Autodesk Inventor part; units mm, degrees
ref_plane "YZ Plane" through (0, 0, 0) normal (1, 0, 0) x (0, 1, 0)
ref_plane "XZ Plane" through (0, 0, 0) normal (0, 1, 0) x (-1, 0, 0)
ref_plane "XY Plane" through (0, 0, 0) normal (0, 0, 1) x (1, 0, 0)
ref_plane "작업 평면1" through (0, 0, 0) normal (0, 0, 1) x (1, 0, 0)
sketch "스케치1" plane through (0, 0, 0) normal (0, 0, 1) x (1, 0, 0)
  line L0 (-85.3, -15) -> (-85.3, -11.5)
  line L1 (-85.3, -15) -> (-79.3, -20.1)
  line L2 (-79.3, -20.1) -> (-26.2, -20.1)
  line L3 (-26.2, -20.1) -> (-20.2, -15)
  line L4 (-20.2, -15) -> (-20.2, 15)
  line L5 (-20.2, 15) -> (-26.2, 20.1)
  line L6 (-26.2, 20.1) -> (-79.3, 20.1)
  line L7 (-79.3, 20.1) -> (-85.3, 15)
  line L8 (-85.3, 11.5) -> (-85.3, 15)
  arc A0 (-82.3, 14.5) -> (-85.3, 11.5) centre (-82.3, 11.5) ccw
  line L9 (-28.8, 14.5) -> (-82.3, 14.5)
  arc A1 (-25.8, 11.5) -> (-28.8, 14.5) centre (-28.8, 11.5) ccw
  line L10 (-25.8, -11.5) -> (-25.8, 11.5)
  arc A2 (-28.8, -14.5) -> (-25.8, -11.5) centre (-28.8, -11.5) ccw
  line L11 (-82.3, -14.5) -> (-28.8, -14.5)
  arc A3 (-85.3, -11.5) -> (-82.3, -14.5) centre (-82.3, -11.5) ccw
  circle A4 centre (-74.8, 17.3) radius 1.35
  circle A5 centre (-52.8, 17.3) radius 1.35
  circle A6 centre (-30.8, 17.3) radius 1.35
  circle A7 centre (-23, 11) radius 1.35
  circle A8 centre (-74.8, -17.3) radius 1.35
  circle A9 centre (-52.8, -17.3) radius 1.35
  circle A10 centre (-30.8, -17.3) radius 1.35
  circle A11 centre (-23, -11) radius 1.35
  line L12 (-15, 14.5) -> (-11.5, 14.5)
  line L13 (-15, 14.5) -> (-20.1, 8.5)
  line L14 (-20.1, 8.5) -> (-20.1, -44.6)
  line L15 (-20.1, -44.6) -> (-15, -50.6)
  line L16 (-15, -50.6) -> (15, -50.6)
  line L17 (15, -50.6) -> (20.1, -44.6)
  line L18 (20.1, -44.6) -> (20.1, 8.5)
  line L19 (20.1, 8.5) -> (15, 14.5)
  line L20 (11.5, 14.5) -> (15, 14.5)
  arc A12 (14.5, 11.5) -> (11.5, 14.5) centre (11.5, 11.5) ccw
  line L21 (14.5, -42) -> (14.5, 11.5)
  arc A13 (11.5, -45) -> (14.5, -42) centre (11.5, -42) ccw
  line L22 (-11.5, -45) -> (11.5, -45)
  arc A14 (-14.5, -42) -> (-11.5, -45) centre (-11.5, -42) ccw
  line L23 (-14.5, 11.5) -> (-14.5, -42)
  arc A15 (-11.5, 14.5) -> (-14.5, 11.5) centre (-11.5, 11.5) ccw
  circle A16 centre (17.3, 4) radius 1.35
  circle A17 centre (17.3, -18) radius 1.35
  circle A18 centre (17.3, -40) radius 1.35
  circle A19 centre (11, -47.8) radius 1.35
  circle A20 centre (-17.3, 4) radius 1.35
  circle A21 centre (-17.3, -18) radius 1.35
  circle A22 centre (-17.3, -40) radius 1.35
  circle A23 centre (-11, -47.8) radius 1.35
  arc A24 (-14.6, -42) -> (-11.5, -45.1) centre (-11.5, -42) ccw
  line L24 (-11.5, -45.1) -> (11.5, -45.1)
  arc A25 (11.5, -45.1) -> (14.6, -42) centre (11.5, -42) ccw
  line L25 (14.6, -42) -> (14.6, 11.5)
  arc A26 (14.6, 11.5) -> (12.5954, 14.4) centre (11.5, 11.5) ccw
  line L26 (12.5954, 14.4) -> (14.9538, 14.4)
  line L27 (14.9538, 14.4) -> (20, 8.4632)
  line L28 (20, 8.4632) -> (20, -44.5632)
  line L29 (14.9538, -50.5) -> (-14.9538, -50.5)
  line L30 (-14.6, 11.5) -> (-14.6, -42)
  arc A27 (-25.7, 11.5) -> (-28.8, 14.6) centre (-28.8, 11.5) ccw
  line L31 (-28.8, 14.6) -> (-82.3, 14.6)
  arc A28 (-82.3, 14.6) -> (-85.2, 12.5954) centre (-82.3, 11.5) ccw
  line L32 (-85.2, 12.5954) -> (-85.2, 14.9538)
  line L33 (-85.2, 14.9538) -> (-79.2632, 20)
  line L34 (-79.2632, 20) -> (-26.2368, 20)
  line L35 (-20.3, -14.9538) -> (-26.2368, -20)
  line L36 (-26.2368, -20) -> (-79.2632, -20)
  line L37 (-79.2632, -20) -> (-85.2, -14.9538)
  line L38 (-85.2, -14.9538) -> (-85.2, -12.5954)
  arc A29 (-85.2, -12.5954) -> (-82.3, -14.6) centre (-82.3, -11.5) ccw
  line L39 (-82.3, -14.6) -> (-28.8, -14.6)
  arc A30 (-28.8, -14.6) -> (-25.7, -11.5) centre (-28.8, -11.5) ccw
  line L40 (-25.7, -11.5) -> (-25.7, 11.5)
  line L41 (-14.6, 15.6629) -> (-14.6, -30)
  circle A31 centre (-23, -11) radius 1.35
  circle A32 centre (-23, 11) radius 1.35
  circle A33 centre (-17.3, -18) radius 1.35
  circle A34 centre (-17.3, 4) radius 1.35
  line L42 (-28.8, 14.6) -> (-54.8, 14.6)
  line L43 (-54.8, 14.6) -> (-54.8, 20)
  line L44 (-54.8, 20) -> (-28.8, 20)
  line L45 (-28.8, 20) -> (-28.8, 14.6)
  line L46 (-28.8, 14.6) -> (-25.7, 14.6)
  line L47 (-28.8, 19.6629) -> (-28.8, 14.6)
  line L48 (-28.8, -14.6) -> (-33.8, -14.6)
  line L49 (-33.8, -14.6) -> (-33.8, -20)
  line L50 (-33.8, -20) -> (-28.8, -20)
  line L51 (-28.8, -20) -> (-28.8, -14.6)
  line L52 (-28.8, -14.6) -> (-25.659, -14.6)
  line L53 (-26.2368, -20) -> (-28.8, -20)
  line L54 (-28.8, -20) -> (-28.8, -14.6)
  line L55 (-14.6, -30) -> (-14.6, -45.1)
  line L56 (-14.6, -50.5) -> (-20, -50.5)
  line L57 (-14.5, -50.5) -> (-7.5, -50.5)
  line L58 (-7.5, -50.5) -> (-7.5, -45.1)
  line L59 (-7.5, -45.1) -> (-14.5, -45.1)
  line L60 (-14.5, -45.1) -> (-14.5, -50.5)
  line L61 (-20, -50.5) -> (-33.8, -20)
  line L62 (-25.659, -14.6) -> (-25.659, 14.6)
  line L63 (-14.5, -45.1) -> (-14.6, -45.1)
  line L64 (-7.5, -45.1) -> (14.9538, -45.1)
  line L65 (14.9538, -45.1) -> (14.9538, -50.5)
  line L66 (14.9538, -50.5) -> (-7.5, -50.5)
  line L67 (-7.5, -50.5) -> (-7.5, -45.1)
  circle A35 centre (11, -47.8) radius 1.35
  line L68 (14.6, -42) -> (20, -42)
  line L69 (20, -42) -> (20, -45.1)
  line L70 (20, -45.1) -> (14.6, -45.1)
  line L71 (14.6, -45.1) -> (14.6, -42)
  line L72 (20, -42) -> (14.6, -42)
  line L73 (14.6, -42) -> (14.6, -38)
  line L74 (14.6, -38) -> (20, -38)
  line L75 (20, -38) -> (20, -42)
  line L76 (20, -45.1) -> (14.9538, -50.5)
  circle A36 centre (-30.8, -17.3) radius 1.35
  circle A37 centre (-17.3, -40) radius 1.35
  circle A38 centre (-11, -47.8) radius 1.35
  circle A39 centre (17.3, -40) radius 1.35
  line L77 (-25.7, 14.6) -> (-25.659, 14.6)
  line L78 (-26.2368, 20) -> (-14.6, 15.6629)
  point P0 (0, 0)
  point P1 (-14.6, -30)
  point P2 (-28.8, 14.6)
  point P3 (-28.8, -14.6)
  point P4 (-26.2368, -20)
  point P5 (-26.0824, -20)
  point P6 (-33.7548, -20.1)
  point P7 (16.4054, -48.9466)
  point P8 (20, -44.7176)
  point P9 (-11.5, -45.1)
  point P10 (-14.6, -30)
  dimension "d0" = 0.1
  dimension "d1" = 0.1
  dimension "d3" = 2.7
  dimension "d4" = 2.7
  dimension "d5" = 2.7
  dimension "d6" = 2.7
  dimension "d9" = 26
  dimension "d10" = 5
  dimension "d11" = 7
  dimension "d16" = 4
extrude "돌출4" add sketch "스케치1" along normal blind 6 contours L61 L36 L51 L52 L62 L77 L46 L45 L34 L78 L5 L4 L3 L2 | L2 L3 L4 L5 L78 L41 L12 L13 L14 L15 L56 L61 | L49 L39 L51 L36 | L15 L14 L13 L12 L41 L30 L55 L63 L60 L29 L56 | L76 L65 L70 L17 | L60 L59 L24 L58 L29 | L45 L31 L43 L34 | L70 L64 L71 L68 L28 L69 L17 | L29 L58 L24 L64 L65 | L68 L25 L74 L28
fillet "모깎기3" radius 2 2 edges at (-20, -50.5, 3) (14.9538, -50.5, 3)
properties part number "leg_ver2" material "PMMA 플라스틱"
Input: part model. Units: mm. Frame: model coordinates. A direction names the side the tool comes from. Round coordinates to 2 decimals unless told otherwise and drop trailing zeros. Loops run counter-clockwise (first coordinate to the right, second up) from the corner with the lowest first, then second, coordinate; pieces in that order, holes last. Notation, with made-up numbers: (24, 23.25) -> (28, 23.25) arc R24 ccw to (28, 51.25) -> close; hole circle Ø4 at (-5.5, -37.75). An arc over 180 degrees is marked (long way). Write each question's results on one line, items separated by ' | '.
1. Section D-D (y = -40). Return loops of the section in (x, z).
Geometry results:
outline: (-24.75, 0) -> (-18.65, 0) -> (-18.65, 6) -> (-24.75, 6) -> close; (-15.95, 0) -> (-14.6, 0) -> (-14.6, 6) -> (-15.95, 6) -> close; (14.6, 0) -> (15.95, 0) -> (15.95, 6) -> (14.6, 6) -> close; (18.65, 0) -> (20, 0) -> (20, 6) -> (18.65, 6) -> close
2. Section B-B (x = 11). Return loops of the section in (y, z), and give its area (3 significant figures).
Geometry results:
outline: (-50.5, 0) -> (-49.15, 0) -> (-49.15, 6) -> (-50.5, 6) -> close; (-46.45, 0) -> (-45.1, 0) -> (-45.1, 6) -> (-46.45, 6) -> close | area: 16.2 mm2
3. Ray query, line 1 (Y direction, x = -11, z = 1.85); line 2 (Y direction, x = -30.8, z = 3.2); line 3 (Y direction, x = -49.5, z = 4.4). Return the intervals inside material, ascending. Write a range as from..to.
Geometry results:
line 1: -50.5..-49.15, -46.45..-45.1 | line 2: -26.63..-18.65, -15.95..-14.6, 14.6..15.95, 18.65..20 | line 3: 14.6..20
4. Mould query, pull axis X, two halves, no side actions, for faces 4 (the face through (-30, -14.6, 3)), 5 (the face through (18.18, -46.86, 2.96)), 6 (the face through (-32.15, -17.36, 2.96)). Classes: +X half, -X half, draft (parallel to the pull), parting line (faces both ways), or undercut.
Geometry results:
face 4: draft | face 5: +X half | face 6: undercut
5. First-contact query: P1, Ø1.6, axis at x = 17.5, z = 2.5, coming from the +Y side; P2, Ø1.5, axis at x = -46.5, z = 2, coming from the -Y side; P3, Ø1, axis at y = -3, z = 1.5, coming from the +X side. Flat tips, straight axial feed; report the tip coordinate or a pass-through.
Geometry results:
P1: y = -38 | P2: y = 14.6 | P3: x = -14.6
6. Set-up query: faces 1 (the face through (-11.176, -49.139, 2.958)), 2 (the face through (17, -38, 3)), 3 (the face through (-33.8, -17, 3)). Return all of +Z, -Z, +X, -X, +Y, -Y with unobstructed straight access to the full face (end or side cutting, diameter ignored); none if empty.
Geometry results:
face 1: +Z, -Z | face 2: +Z, -Z, +X, +Y | face 3: +Z, -Z, -X, -Y
7. Section A-A (y = -11). Return loops of the section in (x, z).
Geometry results:
outline: (-25.66, 0) -> (-24.35, 0) -> (-24.35, 6) -> (-25.66, 6) -> close; (-21.65, 0) -> (-14.6, 0) -> (-14.6, 6) -> (-21.65, 6) -> close
8. Section C-C (z = 3.15). State how many separate pieces and enclosed holes the cut face has, and give its area (3 significant figures).
Geometry results:
separate pieces: 1 | enclosed holes: 11 | area: 1,140 mm2
